```python
from build123d import *

# Parameters (mm, degrees)
SKETCH1_W                                     = 120
SKETCH1_H                                     = 34
BOSS_EXTRUDE1_DEPTH                           = 5
BOSS_EXTRUDE2_DEPTH                           = 9
SKETCH3_R                                     = 6
BOSS_EXTRUDE3_DEPTH                           = 16
CUT_EXTRUDE1_DEPTH                            = 9
SKETCH5_W                                     = 1
SKETCH5_H                                     = 12
CUT_EXTRUDE2_DEPTH                            = 8.5
CBORE_START                                   = 19
CBORE_FOR_M2_HEX_SOCKET_HEAD_CAP_SCREW1_DEPTH = 3.691221609
CBORE_START_2                                 = 17.5
CBORE_FOR_M2_HEX_SOCKET_HEAD_CAP_SCR_3_O_R    = 1.1
CBORE_FOR_M2_HEX_SOCKET_HEAD_CAP_SCR_3_DEPTH  = 1.5
M2_TAPPED_HOLE1_D                             = 1.6
FILLET1_R                                     = 0.2
SKETCH12_W                                    = 120
SKETCH12_H                                    = 34
SKETCH12_R                                    = 14
CUT_EXTRUDE3_DEPTH                            = 10
CUT_EXTRUDE4_DEPTH                            = 83.316462545
CUT_EXTRUDE4_DEPTH_BACK                       = 83.316462545
SKETCH13_W                                    = 2.5
SKETCH13_H                                    = 28
M3_CLEARANCE_HOLE1_D                          = 3.4
M3_CLEARANCE_HOLE1_DEPTH                      = 15
M3_CLEARANCE_HOLE1_TIP                        = 1.021463052


# Read off the part's stored shape, not the designer's step: CBORE for M2 Hex Socket Head Cap Screw1
with BuildPart() as part:
    # Sketch1 → Boss-Extrude1 (new body)
    with BuildSketch(Plane(origin=(0, 0, 0), x_dir=(0, 0, -1), z_dir=(1, 0, 0))):
        with Locations((-60, 17)):
            Rectangle(SKETCH1_W, SKETCH1_H)
    extrude(amount=BOSS_EXTRUDE1_DEPTH)

    # Sketch2 → Boss-Extrude2 (add)
    with BuildSketch(Plane(origin=(5, 0, 0), x_dir=(0, 0, -1), z_dir=(1, 0, 0))):
        with BuildLine():
            ThreePointArc((-52.5, 17), (-54.696699141, 22.303300859), (-60, 24.5))
            Line((-60, 24.5), (-60, 9.5))
            ThreePointArc((-60, 9.5), (-54.696699141, 11.696699141), (-52.5, 17))
        make_face()
        with BuildLine():
            Line((-60, 9.5), (-60, 24.5))
            ThreePointArc((-60, 24.5), (-67.5, 17), (-60, 9.5))
        make_face()
    extrude(amount=BOSS_EXTRUDE2_DEPTH)

    # Sketch3 → Boss-Extrude3 (add)
    with BuildSketch(Plane(origin=(14, 0, 0), x_dir=(0, 0, -1), z_dir=(1, 0, 0))):
        with Locations((-60, 17)):
            Circle(SKETCH3_R)
    extrude(amount=BOSS_EXTRUDE3_DEPTH)

    # Sketch4 → Cut-Extrude1 (cut)
    with BuildSketch(Plane(origin=(30, 0, 0), x_dir=(0, 0, -1), z_dir=(1, 0, 0))):
        with BuildLine():
            Line((-62.449489743, 17.5), (-67.449489743, 17.5))
            Line((-67.449489743, 17.5), (-67.449489743, 16.5))
            Line((-67.449489743, 16.5), (-62.449489743, 16.5))
            ThreePointArc((-62.449489743, 16.5), (-57.5, 17), (-62.449489743, 17.5))
        make_face()
    extrude(amount=-CUT_EXTRUDE1_DEPTH, mode=Mode.SUBTRACT)

    # Sketch5 → Cut-Extrude2 (cut)
    with BuildSketch(Plane.XY.offset(66)):
        with Locations((20.5, 17)):
            Rectangle(SKETCH5_W, SKETCH5_H)
    extrude(amount=-CUT_EXTRUDE2_DEPTH, mode=Mode.SUBTRACT)

    # CBORE for M2 Hex Socket Head Cap Scr 2 → CBORE for M2 Hex Socket Head Cap Screw1 (cut)
    with BuildSketch(Plane(origin=(0, 0, 0), x_dir=(1, 0, 0), z_dir=(0, 1, 0)).offset(CBORE_START)):
        with BuildLine():
            Line((25.709160843, -67), (27.054414631, -65.656854249))
            ThreePointArc((27.054414631, -65.656854249), (25.5, -61.9), (23.945585369, -65.656854249))
            Line((23.945585369, -65.656854249), (25.290839157, -67))
            Line((25.290839157, -67), (25.709160843, -67))
        make_face()
    extrude(amount=CBORE_FOR_M2_HEX_SOCKET_HEAD_CAP_SCREW1_DEPTH, mode=Mode.SUBTRACT)

    # CBORE for M2 Hex Socket Head Cap Scr 3 o → CBORE for M2 Hex Socket Head Cap Scr 3 (cut)
    with BuildSketch(Plane(origin=(0, 0, 0), x_dir=(1, 0, 0), z_dir=(0, 1, 0)).offset(CBORE_START_2)):
        with Locations((25.5, -64.1)):
            Circle(CBORE_FOR_M2_HEX_SOCKET_HEAD_CAP_SCR_3_O_R)
    extrude(amount=CBORE_FOR_M2_HEX_SOCKET_HEAD_CAP_SCR_3_DEPTH, mode=Mode.SUBTRACT)

    # M2 Tapped Hole1 (through all)
    with Locations(Plane(origin=(0, 16.5, 0), x_dir=(1, 0, 0), z_dir=(0, 1, 0))):
        with Locations((25.5, -64.1)):
            Hole(M2_TAPPED_HOLE1_D / 2)

    # Fillet1
    fillet1_edges = [part.edges().sort_by_distance(p)[0] for p in [
        (5, 24.5, 60),
        (14, 17, 66),
    ]]
    fillet(fillet1_edges, radius=FILLET1_R)

    # Sketch12 → Cut-Extrude3 (cut)
    with BuildSketch(Plane(origin=(5, 0, 0), x_dir=(0, 0, -1), z_dir=(1, 0, 0))):
        with Locations((-60, 17)):
            Rectangle(SKETCH12_W, SKETCH12_H)
        with Locations((-60, 17)):
            Circle(SKETCH12_R, mode=Mode.SUBTRACT)
    extrude(amount=-CUT_EXTRUDE3_DEPTH, mode=Mode.SUBTRACT)

    # Sketch13 → Cut-Extrude4 (cut, two sides: drawn at the far end of the back side and taken through both)
    with BuildSketch(Plane(origin=(0, 23, 0), x_dir=(1, 0, 0), z_dir=(0, 1, 0)).offset(-CUT_EXTRUDE4_DEPTH_BACK)):
        with Locations((1.25, -60)):
            Rectangle(SKETCH13_W, SKETCH13_H)
    extrude(amount=CUT_EXTRUDE4_DEPTH + CUT_EXTRUDE4_DEPTH_BACK, mode=Mode.SUBTRACT)

    # M3 Clearance Hole1
    with Locations(Plane(origin=(5, 0, 0), x_dir=(0, 0, -1), z_dir=(1, 0, 0))):
        with Locations((-60, 27.8), (-49.2, 17), (-60, 6.2), (-70.8, 17)):
            Hole(M3_CLEARANCE_HOLE1_D / 2, depth=M3_CLEARANCE_HOLE1_DEPTH)
            with Locations((0, 0, -(M3_CLEARANCE_HOLE1_DEPTH + M3_CLEARANCE_HOLE1_TIP / 2))):  # 118° drill point
                Cone(0, M3_CLEARANCE_HOLE1_D / 2, M3_CLEARANCE_HOLE1_TIP, mode=Mode.SUBTRACT)


solid = part.part
```
Could you check a few things on this model? Use its own coordinates, in mm. A direction names the side the tool comes from. Give positions to 0.01 mm unless a question says otherwise; leave off trailing zeros. Order: outer loops, then holes, each group sorted by start corner. A loop starts at its lowest first (then second) coordinate and runs counter-clockwise, first axis right, second up.
Q1. Suppose I cut it at D-D, the plane x = 13.25. Write out the boundary of the cut face in (y, z).
Q2. I'm going to push flat-ended pins straight in: P1, Ø6, axis at y = 12.5, z = 71, coming from the +X side; P2, Ø7, axis at x = 25.5, z = 64.1, coming from the -Y side; P3, Ø3, axis at x = 27, z = 64.5, coming from the -Y side. Where does each tip first touch, or does it pass through?
Q3. Suppose I cut it at C-C, the plane z = 64.1. Count the separate pieces of the cut face and the enclosed holes in it, and give its area (3 significant figures).
Q4. For faces 1 (the flat face through (14, 23, 63)), 2 (the flat face through (25, 19, 62.9)), 3 (the flat face through (21, 13, 62)), 4 (the cylindrical face through (25.604, 14.714, 63.307)), 5 (the flat face through (26, 16.5, 65)), which set-ups out of +Z, -Z, +X, -X, +Y, -Y let a thin tool reach every point of the face, with its end or its side?
Q5. Suppose I cut it at B-B, the plane x = 25.5. Write out the boundary of the cut face in (y, z).
Q6. If I drill on line 1 along X through (y, z) = (15.5, 64.1); line 2 along Y through (x, z) = (3.45, 60); line 3 along X through (y, z) = (19.9, 64.1), over which ranges is the centre line in solid material (lowest first)?
Q7. We'd pull the mould along Z, two halves only. Please class faces 6 (the cylindrical face through (21.99, 14.7, 54.46)), 7 (the flat face through (5, 11, 54)), 8 (the cylindrical face through (3.73, 17.07, 69.1)): +Z half, -Z half, draft (parallel to the pull), parting line (faces both ways), or undercut.
Q8. Suppose I cut it at A-A, the plane y = 27.8. Write out the boundary of the cut face in (x, z), and give its area (3 significant figures).
Solution:
1. outline: circle Ø15 at (17, 60)
2. P1: stops at x = 5
2. P2: stops at y = 11.03
2. P3: stops at y = 11.8
3. separate pieces: 5
3. enclosed holes: 0
3. area: 282 mm2
4. face 1: +X
4. face 2: +Y
4. face 3: +Z, +Y, -Y
4. face 4: +Y, -Y
4. face 5: +Z, +X
5. outline: (11.99, 63.3) arc R6 ccw (long way) to (22.69, 61.9) - (19, 61.9) - (19, 63) - (17.5, 63) - (17.5, 62.45) arc R2.5 cw (long way) to (16.5, 62.45) - (16.5, 63.3) - close; (13.54, 64.9) - (16.5, 64.9) - (16.5, 65.98) arc R6 ccw to start; (17.5, 65.2) - (19, 65.2) - (19, 65.66) arc R6 ccw to (17.5, 65.98) - close
6. line 1: x = 2.5 to 20, 21 to 24.7, 26.3 to 30
6. line 2: y = 3 to 4.5, 7.9 to 26.1, 29.5 to 31
6. line 3: x = 2.5 to 20, 21 to 23.3, 27.7 to 30
7. face 6: parting line
7. face 7: draft
7. face 8: undercut
8. outline: (2.5, 51.09) - (5, 51.09) - (5, 58.3) - (2.5, 58.3) - close; (2.5, 61.7) - (5, 61.7) - (5, 68.91) - (2.5, 68.91) - close
8. area: 36.0 mm2
